```python
from build123d import *

# Parameters (mm, degrees)
SKETCH001_R     = 3.75
POCKET_DEPTH    = 9.70192
CHAMFER_SIZE    = 0.4
CHAMFER001_SIZE = 0.1


with BuildPart() as pocket:
    # Sketch003 → Revolution001 (revolve)
    with BuildSketch(Plane.XZ):
        Polygon((0, 0.29908), (2.75, 1.3), (2.75, 10), (0, 10), align=None)
    revolve(axis=Axis((0, 0, 0), (0, 0, 1)))

    # Sketch001 → Pocket (cut, through all)
    with BuildSketch(Plane(origin=(0, 0, 10), x_dir=(-1, 0, 0), z_dir=(0, 0, 1))):
        Circle(SKETCH001_R)
        Polygon((-0.721688, 1.25), (0.721688, 1.25), (1.443376, 0), (0.721688, -1.25), (-0.721688, -1.25), (-1.443376, 0), align=None, mode=Mode.SUBTRACT)
    extrude(amount=-POCKET_DEPTH, mode=Mode.SUBTRACT)


with BuildPart() as chamfer001:
    # Sketch → Revolution (revolve)
    with BuildSketch(Plane.XZ):
        Polygon((1.45, 3), (2.75, 3), (2.75, 0), (1.5, 0), (1.5, -22), (0, -22), (0, 1.549999), align=None)
    revolve(axis=Axis((0, 0, 0), (0, 0, 1)))

    # Cut: cut Pocket
    add(pocket.part, mode=Mode.SUBTRACT)

    # Chamfer
    chamfer_edges = [chamfer001.edges().sort_by_distance(p)[0] for p in [
        (-1.5, 0, -22),
    ]]
    chamfer(chamfer_edges, length=CHAMFER_SIZE)

    # Chamfer001
    chamfer001_edges = [chamfer001.edges().sort_by_distance(p)[0] for p in [
        (-2.75, 0, 0),
        (-2.75, 0, 3),
    ]]
    chamfer(chamfer001_edges, length=CHAMFER001_SIZE)


solid = chamfer001.part
```
CAD build for the part. Positions are in the model's coordinates, mm. A direction names the side the tool comes from. Round coordinates to 2 decimals unless told otherwise and drop trailing zeros. Order: outer loops, then holes, each group sorted by start corner. A loop starts at its lowest first (then second) coordinate and runs counter-clockwise, first axis right, second up. Notation, with made-up numbers: (11.5, 33.5) - (21.5, 33.5) arc R18 ccw to (21.5, 43.5) - close; hole circle Ø10 at (35, -18.75). An arc over 180 degrees is marked (long way). Answer in a Markdown table with one row per item. Add a question column.
(1) Drop flat-ended pins along their axis: pin 1 Ø2 at (x, z) = (1, -7) entering from -Y; pin 2 Ø1.5 at (x, z) = (-2, -5) entering from -Y; pin 3 Ø1.5 at (y, z) = (2, -17) entering from +X. Give the stop position or say it passes through.
(2) Mould opens along Y. For faces 4 (the face through (0, -2, 0)), 5 (the face through (1.088, -0.616, 1.889)), 6 (the face through (-0.596, -2.685, 1.48)) say: +Y half, -Y half, draft (parallel to the pull), parting line (faces both ways), or undercut.
(3) Band-saw the part on A-A on z = -16. List the corners of the cut face in (x, y).
(4) 3-axis set-ups, long thin cutter, end or side, ignore diameter. For faces 1 (the face through (-1.5, 0.07, -10.95)), 2 (the face through (-1.14, -1.14, 3)), 3 (the face through (1.08, 0.63, 1.89)): which of +Z, -Z, +X, -X, +Y, -Y reach the whole face in a straight line?
(5) Probe L1, parallel to Z at x = -1.6, y = 1.65; L2, parallel to Z at x = 0.5, y = 0.35; L3, parallel to X at y = 0.15, z = -8.5. List the from-to ranges inside material, lowest first. Write a range as [from, to].
Data:
| question | item | result |
|---|---|---|
| 1 | pin 1 | stops at y = -1.5 |
| 1 | pin 2 | stops at y = -0.83 |
| 1 | pin 3 | stops at x = 0.83 |
| 2 | face 4 | draft |
| 2 | face 5 | undercut |
| 2 | face 6 | parting line |
| 3 | outline | circle Ø3 at (0, 0) |
| 4 | face 1 | -Z |
| 4 | face 2 | +Z, +X, -X, +Y, -Y |
| 4 | face 3 | +Z |
| 5 | L1 | z = [0, 3] |
| 5 | L2 | z = [-22, 0.52] |
| 5 | L3 | x = [-1.49, 1.49] |
